from build123d import *

# Parameters (mm, degrees)
SALIENTE_EXTRUIR1_DEPTH = 40
CROQUIS2_R              = 1.5
CORTAR_EXTRUIR2_DEPTH   = 4.5
CROQUIS3_R              = 11
CROQUIS3_R_2            = 4
SALIENTE_EXTRUIR3_DEPTH = 2
CROQUIS8_R              = 4
SALIENTE_EXTRUIR4_DEPTH = 150
CROQUIS9_W              = 16
CROQUIS9_H              = 10.5
SALIENTE_EXTRUIR6_DEPTH = 6.5


with BuildPart() as part:
    # Croquis1 → Saliente-Extruir1 (new body)
    with BuildSketch(Plane(origin=(0, 0, 0), x_dir=(1, 0, 0), z_dir=(0, 1, 0))):
        Polygon((-18.15, -21.15), (18.15, -21.15), (21.15, -18.15), (21.15, 18.15), (18.15, 21.15), (-18.15, 21.15), (-21.15, 18.15), (-21.15, -18.15), align=None)
    extrude(amount=SALIENTE_EXTRUIR1_DEPTH)

    # Croquis2 → Cortar-Extruir2 (cut)
    with BuildSketch(Plane(origin=(0, 40, 0), x_dir=(1, 0, 0), z_dir=(0, 1, 0))):
        with Locations(Location((15.05, 15.05, 0), (0, 0, 270))):
            Circle(CROQUIS2_R)
        with Locations(Location((-15.95, 15.05, 0), (0, 0, 270))):
            Circle(CROQUIS2_R)
        with Locations(Location((-15.95, -15.95, 0), (0, 0, 270))):
            Circle(CROQUIS2_R)
        with Locations(Location((15.05, -15.95, 0), (0, 0, 270))):
            Circle(CROQUIS2_R)
    extrude(amount=-CORTAR_EXTRUIR2_DEPTH, mode=Mode.SUBTRACT)

    # Croquis3 → Saliente-Extruir3 (add)
    with BuildSketch(Plane(origin=(0, 40, 0), x_dir=(1, 0, 0), z_dir=(0, 1, 0))):
        with Locations(Location((0, 0, 0), (0, 0, 90))):
            Circle(CROQUIS3_R)
        with Locations(Location((0, 0, 0), (0, 0, 270))):
            Circle(CROQUIS3_R_2, mode=Mode.SUBTRACT)
    extrude(amount=SALIENTE_EXTRUIR3_DEPTH)

    # Croquis8 → Saliente-Extruir4 (add)
    with BuildSketch(Plane(origin=(0, 40, 0), x_dir=(1, 0, 0), z_dir=(0, 1, 0))):
        with Locations(Location((0, 0, 0), (0, 0, 270))):
            Circle(CROQUIS8_R)
    extrude(amount=SALIENTE_EXTRUIR4_DEPTH)

    # Croquis9 → Saliente-Extruir6 (add)
    with BuildSketch(Plane.XY.offset(21.15)):
        with Locations((0, 5.25)):
            Rectangle(CROQUIS9_W, CROQUIS9_H)
    extrude(amount=SALIENTE_EXTRUIR6_DEPTH)


solid = part.part
Can you work these out from the model? Positions are in its coordinate system, mm. A direction names the side the tool comes from. Coordinates: 2 decimals unless noted, no trailing zeros. Write each loop counter-clockwise with the first axis right and the second up, starting at its lowest first coordinate (ties: lowest second). Pieces come first, ordered by that corner, then holes. Notation, with made-up numbers: (-21, 39.5) -> (5, 39.5) arc R13 cw to (5, 63.5) -> close; hole circle Ø10 at (55.25, 18.25). An arc over 180 degrees is marked (long way). Write each question's results on one line, items separated by ' | '. Start each with the question number.
Item 1: On a 3-axis mill with a long thin cutter (end or side, diameter ignored), from which of +Z, -Z, +X, -X, +Y, -Y can I reach the whole of each face in a straight line? I mean faces 1 (the flat face through (-8, 5, 24)), 2 (the cylindrical face through (10.74, 40.99, 2.38)), 3 (the flat face through (8, 5, 24)). Say none if no direction works.
Item 2: If we section it at A-A, the plane x = 0: Write out the boundary of the cut face in (y, z).
Item 3: If we section it at B-B, the plane z = 0: Write out the boundary of the cut face in (x, y).
Item 4: I'm going to push flat-ended pins straight in: P1, Ø4, axis at x = -15.95, z = -15.05, coming from the +Y side; P2, Ø1.5, axis at x = -16.5, z = -15.5, coming from the +Y side; P3, Ø3, axis at y = 3, z = 25, coming from the -X side. Where does each tip first touch, or does it pass through?
Item 5: Please list where these lines run through material, in increasing order: probe 1 along X at (y, z) = (38.3, 15.95); probe 2 along Y at (x, z) = (2.5, -15); probe 3 along Y at (x, z) = (4, 25).
Item 6: If we section it at C-C, the plane y = 176: Write out the boundary of the cut face in (x, z), and give its area (3 significant figures).
Answer block:
1) face 1: +Z, -X, +Y, -Y | face 2: +Y | face 3: +Z, +X, +Y, -Y
2) outline: (0, -21.15) -> (40, -21.15) -> (40, -11) -> (42, -11) -> (42, -4) -> (190, -4) -> (190, 4) -> (42, 4) -> (42, 11) -> (40, 11) -> (40, 21.15) -> (10.5, 21.15) -> (10.5, 27.65) -> (0, 27.65) -> close
3) outline: (-21.15, 0) -> (21.15, 0) -> (21.15, 40) -> (11, 40) -> (11, 42) -> (4, 42) -> (4, 190) -> (-4, 190) -> (-4, 42) -> (-11, 42) -> (-11, 40) -> (-21.15, 40) -> close
4) P1: y = 40 | P2: y = 35.5 | P3: x = -8
5) probe 1: -21.15 to -17.45, -14.45 to 13.55, 16.55 to 21.15 | probe 2: 0 to 40 | probe 3: 0 to 10.5
6) outline: circle Ø8 at (0, 0) | area: 50.3 mm²
